Autodesk Inventor part; units mm, degrees
ref_plane "YZ Plane" through (0, 0, 0) normal (1, 0, 0) x (0, 1, 0)
ref_plane "XZ Plane" through (0, 0, 0) normal (0, 1, 0) x (-1, 0, 0)
ref_plane "XY Plane" through (0, 0, 0) normal (0, 0, 1) x (1, 0, 0)
sketch "Sketch1" plane through (0, 0, 0) normal (0, 1, 0) x (-1, 0, 0)
  circle A0 centre (0, 0) radius 50
  circle A1 centre (0, 0) radius 45
  line L0 (5, 48.7261) -> (-5, 48.7261)
  line L1 (-5, 48.7261) -> (-5, -48.4617)
  line L2 (-5, -48.4617) -> (5, -48.4617)
  line L3 (5, -48.4617) -> (5, 48.7261)
  line L4 (48.4415, 5) -> (-48.0304, 5)
  line L5 (-48.0304, 5) -> (-48.0304, -5)
  line L6 (-48.0304, -5) -> (48.4415, -5)
  line L7 (48.4415, -5) -> (48.4415, 5)
  dimension "d0" = 100
  dimension "d1" = 90
  dimension "d2" = 5
  dimension "d3" = 5
  dimension "d4" = 5
  dimension "d5" = 5
extrude "Extrusion1" add sketch "Sketch1" along normal blind 3 contours A0 | A1 L6 L3 L4 | A1 L4 L7 L6 | L3 L4 L1 A1 | A1 L1 L0 L3 | L3 L6 L1 L4 | L3 L2 L1 A1 | A1 L1 L6 L3 | L1 L6 A1 L4 | A1 L6 L5 L4
sketch "Sketch2" plane through (0, 3, 0) normal (0, 1, 0) x (1, 0, 0)
  circle A0 centre (0, 0) radius 40
  circle A1 centre (0, 0) radius 37.5
  circle A2 centre (0, 0) radius 25
  circle A3 centre (0, 0) radius 22.5
  dimension "d8" = 80
  dimension "d9" = 75
  dimension "d10" = 50
  dimension "d11" = 45
extrude "Extrusion2" add sketch "Sketch2" against normal blind 3
sketch "Sketch3" plane through (0, 3, 0) normal (0, 1, 0) x (1, 0, 0)
  circle A0 centre (0, 0) radius 4.5
  line L0 (-1.51, -3.1) -> (1.69, -3.1)
  line L1 (1.69, -3.1) -> (1.69, 3.1)
  line L2 (1.69, 3.1) -> (-1.51, 3.1)
  line L3 (-1.51, 3.1) -> (-1.51, -3.1)
  dimension "d14" = 9
  dimension "d15" = 6.2
  dimension "d16" = 3.2
  dimension "d17" = 1.51
  dimension "d18" = 3.1
extrude "Extrusion3" add sketch "Sketch3" along normal blind 7
sketch "Sketch4" plane through (0, 3, 0) normal (0, 1, 0) x (1, 0, 0)
  point P0 (0, 0)
sketch "Sketch5" plane through (0, 0, 0) normal (0, -1, 0) x (1, 0, 0)
  line L0 (45, 3) -> (-45, 3)
  line L1 (-45, 3) -> (-45, -3)
  line L2 (-45, -3) -> (45, -3)
  line L3 (45, -3) -> (45, 3)
  line L4 (3, 45) -> (-3, 45)
  line L5 (-3, 45) -> (-3, -45)
  line L6 (-3, -45) -> (3, -45)
  line L7 (3, -45) -> (3, 45)
  point P0 (0, 0)
  dimension "d21" = 90
  dimension "d22" = 90
  dimension "d23" = 45
  dimension "d24" = 45
  dimension "d25" = 3
  dimension "d26" = 3
  dimension "d27" = 3
  dimension "d28" = 3
extrude "Extrusion4" cut sketch "Sketch5" against normal blind 3
sketch "Sketch6" plane through (0, 0, 0) normal (0, -1, 0) x (1, 0, 0)
  line L0 (5.0041, 4.9106) -> (-5, 4.9106)
  line L1 (-5, 4.9106) -> (-5, -5)
  line L2 (-5, -5) -> (5.0041, -5)
  line L3 (5.0041, -5) -> (5.0041, 4.9106)
  point P0 (0, 0)
extrude "Extrusion5" add sketch "Sketch6" against normal blind 3
fillet "Fillet1" radius 2 8 edges at (3, 1.5, 4.9106) (-3, 1.5, 4.9106) (-5, 1.5, 3) (-5, 1.5, -3) (-3, 1.5, -5) (3, 1.5, -5) (5.0041, 1.5, -3) (5.0041, 1.5, 3)
fillet "Fillet2" radius 2 8 edges at (45, 1.5, 3) (45, 1.5, -3) (3, 1.5, 45) (-3, 1.5, 45) (-45, 1.5, 3) (-45, 1.5, -3) (-3, 1.5, -45) (3, 1.5, -45)
properties part number "Scanning Disk"
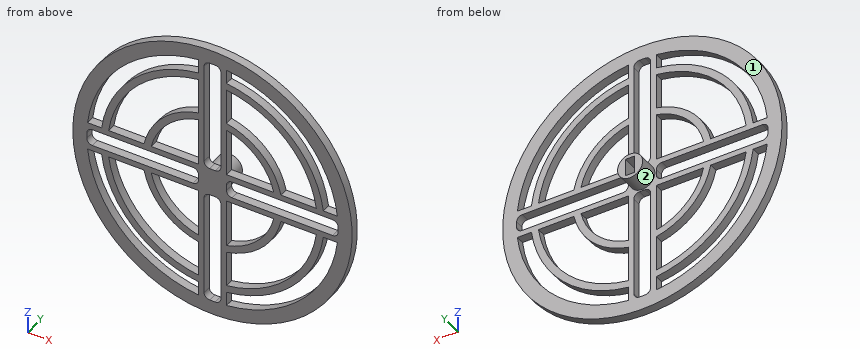
The model under review builds one solid part; all positions refer to its coordinate system, in mm. Face numbers are marked on the shaded views. Round coordinates to 2 decimals unless told otherwise and drop trailing zeros. Loops run counter-clockwise (first coordinate to the right, second up) from the corner with the lowest first, then second, coordinate; pieces in that order, holes last. Notation, with made-up numbers: (83.25, 75) -> (139.25, 75) arc R26 cw to (139.25, 96) -> close; hole circle Ø3 at (84, 56.5). An arc over 180 degrees is marked (long way). Answer in a Markdown table with one row per item.
1) Wall thickness on line 1 along Z through (x, y) = (-41.5, 1.5); line 2 along Y through (x, z) = (39, -4); line 3 along X through (y, z) = (0.5, 22): over which ranges is each line inside the solid? List them lowest first.
Taken from the geometry:
| item | result |
|---|---|
| line 1 | z = -27.89 to -17.4, -5 to -3, 3 to 5, 17.4 to 27.89 |
| line 2 | y = 0 to 3 |
| line 3 | x = -44.9 to -39.26, -33.41 to -30.37, -11.87 to -3, 3 to 11.87, 30.37 to 33.41, 39.26 to 44.9 |
2) Draft analysis for pull direction Z (two halves, no side actions). For the marked faces 1 and 2, state which applies: pulls with the +Z half, pulls with the -Z half, needs draft (parallel to the pull), parting line crosses it, or undercut.
Taken from the geometry:
| item | result |
|---|---|
| face 1 | needs draft |
| face 2 | parting line crosses it |
3) Consider section A-A, the plane z = 29.5. Write out the cut boundary in (x, y), plus the area to 3 significant figures.
Taken from the geometry:
| item | result |
|---|---|
| outline | (-40.37, 0) -> (-33.98, 0) -> (-33.98, 3) -> (-40.37, 3) -> close; (-27.01, 0) -> (-23.15, 0) -> (-23.15, 3) -> (-27.01, 3) -> close; (-5, 0) -> (-3, 0) -> (-3, 3) -> (-5, 3) -> close; (3, 0) -> (5, 0) -> (5, 3) -> (3, 3) -> close; (23.15, 0) -> (27.01, 0) -> (27.01, 3) -> (23.15, 3) -> close; (33.98, 0) -> (40.37, 0) -> (40.37, 3) -> (33.98, 3) -> close |
| area | 73.5 mm² |
4) Consider section C-C, the plane x = 9.5. Count the separate pieces of the cut face and the enclosed holes in it, plus the area to 3 significant figures.
Taken from the geometry:
| item | result |
|---|---|
| separate pieces | 8 |
| enclosed holes | 0 |
| area | 74.5 mm² |
5) Consider section D-D, the plane y = 5. Write out the cut boundary in (x, z), plus the area to 3 significant figures.
Taken from the geometry:
| item | result |
|---|---|
| outline | circle Ø9 at (0, 0); hole (-1.51, -3.1) -> (1.69, -3.1) -> (1.69, 3.1) -> (-1.51, 3.1) -> close |
| area | 43.8 mm² |
6) Consider section B-B, the plane x = -32. Write out the cut boundary in (y, z).
Taken from the geometry:
| item | result |
|---|---|
| outline | (0, -38.42) -> (3, -38.42) -> (3, -31.64) -> (0, -31.64) -> close; (0, -24) -> (3, -24) -> (3, -19.55) -> (0, -19.55) -> close; (0, -5) -> (3, -5) -> (3, -3) -> (0, -3) -> close; (0, 3) -> (3, 3) -> (3, 5) -> (0, 5) -> close; (0, 19.55) -> (3, 19.55) -> (3, 24) -> (0, 24) -> close; (0, 31.64) -> (3, 31.64) -> (3, 38.42) -> (0, 38.42) -> close |
7) For pin 1 Ø0.9 at (y, z) = (1, 42.5) entering from +X; pin 2 Ø2.5 at (x, y) = (-15, 1) entering from +Z; pin 3 Ø0.9 at (y, z) = (1.5, 10.5) entering from -X; pin 4 Ø1 at (x, z) = (21, -12.5) entering from -Y, all flat-tipped, find the tip position at first contact; note any pin that passes through.
Taken from the geometry:
| item | result |
|---|---|
| pin 1 | stops at x = 27.05 |
| pin 2 | stops at z = 48.07 |
| pin 3 | stops at x = -48.98 |
| pin 4 | stops at y = 0 |
